Read the model definition and answer for the solid it produces. Units are mm, in the model's axes. Coordinates: 2 decimals unless noted, no trailing zeros. Order: outer loops, then holes, each group sorted by start corner. A loop starts at its lowest first (then second) coordinate and runs counter-clockwise, first axis right, second up. Notation, with made-up numbers: (26.25, 88.5) - (84.25, 88.5) arc R26 ccw to (84.25, 120.5) - close; hole circle Ø10 at (57, 45). An arc over 180 degrees is marked (long way). Write item = value, one per line.
from build123d import *

# Parameters (mm, degrees)
SKETCH1_R           = 7.5
BOSS_EXTRUDE1_DEPTH = 10
FILLET1_R           = 5


with BuildPart() as part:
    # Sketch1 → Boss-Extrude1 (new body)
    with BuildSketch(Plane.XY):
        with BuildLine():
            Line((175, 20), (13.900856021, 58.367509814))
            ThreePointArc((13.900856021, 58.367509814), (-60, 0), (13.900856021, -58.367509814))
            Line((13.900856021, -58.367509814), (175, -20))
            ThreePointArc((175, -20), (195, 0), (175, 20))
        make_face()
        with Locations((175, 0)):
            Circle(SKETCH1_R, mode=Mode.SUBTRACT)
        Polygon((40.5, 23.382685902), (0, 46.765371804), (-40.5, 23.382685902), (-40.5, -23.382685902), (0, -46.765371804), (40.5, -23.382685902), align=None, mode=Mode.SUBTRACT)
    extrude(amount=BOSS_EXTRUDE1_DEPTH)

    # Fillet1
    fillet1_edges = [part.edges().sort_by_distance(p)[0] for p in [
        (0, -46.765371804, 5),
        (40.5, -23.382685902, 5),
        (40.5, 23.382685902, 5),
        (0, 46.765371804, 5),
        (-40.5, 23.382685902, 5),
        (-40.5, -23.382685902, 5),
    ]]
    fillet(fillet1_edges, radius=FILLET1_R)


solid = part.part
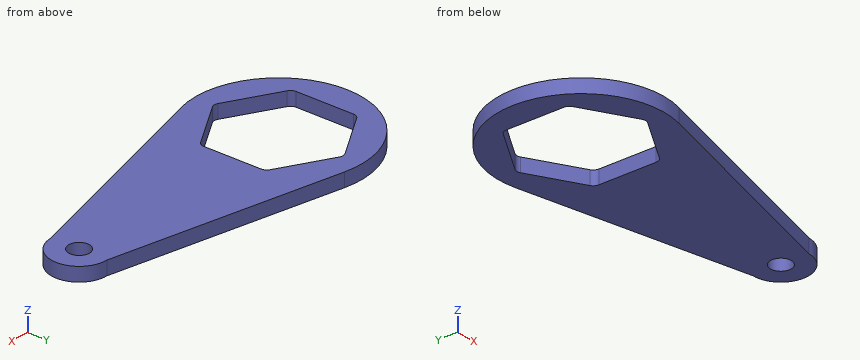
1) The part is cut by section A-A (z = 3.75). Determine the outline of the cut face in (x, y), and give its area (3 significant figures).
Returned:
outline = (13.9, -58.37) - (175, -20) arc R20 ccw to (175, 20) - (13.9, 58.37) arc R60 ccw (long way) to start; hole (-40.5, -20.5) arc R5 ccw to (-38, -24.83) - (-2.5, -45.32) arc R5 ccw to (2.5, -45.32) - (38, -24.83) arc R5 ccw to (40.5, -20.5) - (40.5, 20.5) arc R5 ccw to (38, 24.83) - (2.5, 45.32) arc R5 ccw to (-2.5, 45.32) - (-38, 24.83) arc R5 ccw to (-40.5, 20.5) - close; hole circle Ø15 at (175, 0)
area = 14,700 mm^2
2) Straight lines are drawn through the part: line 1 along Y through (x, z) = (175, 5.75); line 2 along X through (y, z) = (6, 9); line 3 along X through (y, z) = (-17, 8.5). For each, find the intervals that lie inside material, in ascending order. Write a range as from..to.
Returned:
line_1 = -20..-7.5, 7.5..20
line_2 = -59.7..-40.5, 40.5..170.5, 179.5..194.08
line_3 = -57.54..-40.5, 40.5..185.54
3) The part is cut by section D-D (y = -40). Determine the outline of the cut face in (x, z).
Returned:
outline = (-44.72, 0) - (-11.72, 0) - (-11.72, 10) - (-44.72, 10) - close; (11.72, 0) - (91.02, 0) - (91.02, 10) - (11.72, 10) - close
4) The part is cut by section B-B (x = 0). Determine the outline of the cut face in (y, z).
Returned:
outline = (-60, 0) - (-45.99, 0) - (-45.99, 10) - (-60, 10) - close; (45.99, 0) - (60, 0) - (60, 10) - (45.99, 10) - close
5) The part is cut by section C-C (y = 4.5). Determine the outline of the cut face in (x, z).
Returned:
outline = (-59.83, 0) - (-40.5, 0) - (-40.5, 10) - (-59.83, 10) - close; (40.5, 0) - (169, 0) - (169, 10) - (40.5, 10) - close; (181, 0) - (194.49, 0) - (194.49, 10) - (181, 10) - close
6) Flat-ended cylindrical pins translate along their axes: pin 1 Ø5 at (x, z) = (169, 3.5) entering from -Y; pin 2 Ø4 at (x, z) = (149.5, 9) entering from +Y; pin 3 Ø4 at (x, z) = (84, 3.5) entering from +Y. Find the tip coordinate at first contact, or state that the pin passes through.
Returned:
pin_1 = -22.02
pin_2 = 26.55
pin_3 = 42.15
